Autodesk Inventor part; units mm, degrees
ref_plane "YZ Plane" through (0, 0, 0) normal (1, 0, 0) x (0, 1, 0)
ref_plane "XZ Plane" through (0, 0, 0) normal (0, 1, 0) x (-1, 0, 0)
ref_plane "XY Plane" through (0, 0, 0) normal (0, 0, 1) x (1, 0, 0)
sketch "Sketch1" plane through (0, 0, 0) normal (0, 0, 1) x (1, 0, 0)
  circle A0 centre (0, 0) radius 107.95
  circle A1 centre (0, 0) radius 114.3
  circle A2 centre (0, 0) radius 107.95
  circle A3 centre (0, 0) radius 107.95
  line L0 (-63.5, -63.5) -> (63.5, -63.5)
  line L1 (63.5, -63.5) -> (63.5, 63.5)
  line L2 (63.5, 63.5) -> (-63.5, 63.5)
  line L3 (-63.5, 63.5) -> (-63.5, -63.5)
  line L4 (-63.5, -63.5) -> (63.5, 63.5) construction
  line L5 (63.5, -63.5) -> (-63.5, 63.5) construction
  line L6 (57.15, 57.15) -> (57.15, -57.15)
  line L7 (57.15, -57.15) -> (-57.15, -57.15)
  line L8 (-57.15, -57.15) -> (-57.15, 57.15)
  line L9 (-57.15, 57.15) -> (57.15, 57.15)
  dimension "d0" = 127
  dimension "d1" = 127
  dimension "d2" = 6.35
extrude "Extrusion1" add sketch "Sketch1" along normal blind 6.35 contours L3 L2 L1 L0 | L6 L7 L8 L9
sketch "Sketch2" plane through (0, 0, 6.35) normal (0, 0, 1) x (1, 0, 0)
  line L0 (63.5, -63.5) -> (63.5, 63.5)
  line L1 (-63.5, 63.5) -> (63.5, 63.5)
  line L2 (63.5, 63.5) -> (63.5, -63.5)
  line L3 (63.5, -63.5) -> (-63.5, -63.5)
  line L4 (-63.5, -63.5) -> (-63.5, 63.5)
  line L5 (-63.5, 63.5) -> (63.5, -63.5) construction
  line L6 (63.5, 63.5) -> (-63.5, -63.5) construction
  line L7 (-57.15, -57.15) -> (57.15, -57.15)
  line L8 (57.15, -57.15) -> (57.15, 57.15)
  line L9 (57.15, 57.15) -> (-57.15, 57.15)
  line L10 (-57.15, 57.15) -> (-57.15, -57.15)
  point P0 (0, 0)
  dimension "d5" = 6.35
extrude "Extrusion2" add sketch "Sketch2" along normal blind 152.4
sketch "Sketch3" plane through (-63.5, -63.5, 0) normal (-1, 0, 0) x (0, 0, 1)
  line L0 (0, 127) -> (0, 0)
  line L1 (0, 0) -> (158.75, 0)
  line L2 (158.75, 127) -> (158.75, 0)
  line L3 (0, 127) -> (158.75, 127)
  point P0 (0, 63.5)
extrude "Extrusion3" add sketch "Sketch3" along normal blind 19.05
sketch "Sketch4" plane through (-82.55, -63.5, 0) normal (-1, 0, 0) x (0, 0, 1)
  line L0 (107.95, 6.35) -> (146.05, 6.35)
  line L1 (146.05, 6.35) -> (146.05, 120.65)
  line L2 (146.05, 120.65) -> (107.95, 120.65)
  line L3 (107.95, 120.65) -> (107.95, 6.35)
  line L4 (107.95, 6.35) -> (146.05, 120.65) construction
  line L5 (146.05, 6.35) -> (107.95, 120.65) construction
  line L6 (158.75, 127) -> (0, 127)
  line L7 (0, 0) -> (158.75, 0)
  line L8 (158.75, 0) -> (158.75, 127)
  point P0 (0, 63.5)
  point P1 (127, 63.5)
  dimension "d10" = 38.1
  dimension "d11" = 114.3
  dimension "d12" = 6.35
  dimension "d13" = 6.35
  dimension "d14" = 12.7
extrude "Extrusion4" cut sketch "Sketch4" against normal blind 7.62
ref_plane "Work Plane1" through (0, 0, 25.4) normal (0, 0, 1) x (1, 0, 0)
sketch "Sketch6" plane through (0, 0, 25.4) normal (0, 0, 1) x (1, 0, 0)
  line L0 (-57.15, -57.15) -> (57.15, -57.15)
  line L1 (57.15, -57.15) -> (57.15, 57.15)
  line L2 (57.15, 57.15) -> (-57.15, 57.15)
  line L3 (-57.15, 57.15) -> (-57.15, -57.15)
  point P0 (0, 0)
extrude "Extrusion5" add sketch "Sketch6" along normal blind 6.35
sketch "Sketch7" plane through (63.5, 63.5, 158.75) normal (0, 1, 0) x (1, 0, 0)
  line L0 (-6.35, 133.35) -> (-120.65, 133.35)
  line L1 (-120.65, 127) -> (-6.35, 127)
  circle A0 centre (-19.05, 122.0738) radius 3.175
  circle A1 centre (-43.18, 122.0738) radius 3.175
  circle A2 centre (-67.31, 122.0738) radius 3.175
  circle A3 centre (-91.44, 122.0738) radius 3.175
  circle A4 centre (-115.57, 122.0738) radius 3.175
  line L2 (-15.875, 122.0738) -> (-22.225, 122.0738)
  line L3 (-40.005, 122.0738) -> (-46.355, 122.0738)
  line L4 (-64.135, 122.0738) -> (-70.485, 122.0738)
  line L5 (-88.265, 122.0738) -> (-94.615, 122.0738)
  line L6 (-112.395, 122.0738) -> (-118.745, 122.0738)
  point P0 (-63.5, 158.75)
  dimension "d20" = 6.35
  dimension "d21" = 12.7
  dimension "d24" = 24.13
extrude "Extrusion6" cut sketch "Sketch7" against normal blind 127 contours L2 A0 | L3 A1 | L4 A2 | L5 A3 | L6 A4 picked at (-18.2578, 122.7756) picked at (-43.0524, 123.1244) picked at (-66.7088, 122.9448) picked at (-90.8388, 122.9448) picked at (-114.8476, 123.4366)
sketch "Sketch8" plane through (63.5, -63.5, 0) normal (1, 0, 0) x (0, 0, -1)
  line L0 (-6.35, 120.65) -> (-25.4, 120.65)
  line L1 (-158.75, 6.35) -> (-6.35, 6.35)
  line L2 (-6.35, 120.65) -> (-158.75, 120.65)
  line L3 (-6.35, 120.65) -> (-6.35, 6.35)
  line L4 (-6.35, 6.35) -> (-6.35, 120.65)
  line L5 (-28.575, 6.35) -> (-28.575, 120.65)
  point P0 (0, 63.5)
  point P1 (-25.4, 6.35)
extrude "Extrusion7" cut sketch "Sketch8" against normal blind 6.35
sketch "Sketch9" plane through (-57.15, 57.15, 6.35) normal (0, -1, 0) x (1, 0, 0)
  circle A0 centre (117.475, 19.05) radius 2.033
  line L0 (114.3, 19.05) -> (0, 19.05)
  line L1 (0, 0) -> (0, 19.05)
  line L2 (120.65, 0) -> (0, 0)
  line L3 (120.65, 22.225) -> (120.65, 0)
  line L4 (120.65, 22.225) -> (114.3, 22.225)
  line L5 (114.3, 22.225) -> (114.3, 19.05)
  point P0 (57.15, -6.35)
  dimension "d34" = 3.175
  dimension "d35" = 3.175
extrude "Extrusion8" cut sketch "Sketch9" along normal mid plane 254 contours A0
sketch "Sketch10" plane through (0, 0, 0) normal (0, 0, -1) x (-1, 0, 0)
  line L0 (57.15, 57.15) -> (57.15, -57.15)
  line L1 (74.93, -57.15) -> (74.93, 57.15)
  line L2 (57.15, 57.15) -> (74.93, 57.15)
  line L3 (82.55, -57.15) -> (74.93, -57.15)
  line L4 (57.15, -57.15) -> (74.93, -57.15)
  line L5 (60.325, 57.15) -> (60.325, -57.15)
  point P0 (0, 0)
  dimension "d40" = 3.175
extrude "Extrusion9" cut sketch "Sketch10" against normal blind 114.3 contours L2 L1 L4 L5
sketch "Sketch11" plane through (-82.55, -63.5, 0) normal (-1, 0, 0) x (0, 0, 1)
  line L0 (6.35, 120.65) -> (6.35, 6.35)
  line L1 (6.35, 120.65) -> (6.35, 6.35)
  line L2 (25.4, 120.65) -> (25.4, 6.35)
  line L3 (6.35, 6.35) -> (25.4, 6.35)
  line L4 (6.35, 120.65) -> (25.4, 120.65)
  line L5 (25.4, 120.65) -> (6.35, 120.65)
  point P0 (0, 63.5)
extrude "Extrusion10" cut sketch "Sketch11" against normal blind 42.8625
sketch "Sketch12" plane through (-60.325, -57.15, 0) normal (-1, 0, 0) x (0, 0, 1)
  point P0 (0, 57.15)
sketch "Sketch13" plane through (-60.325, -57.15, 0) normal (-1, 0, 0) x (0, 0, 1)
  line L0 (0, 114.3) -> (6.35, 114.3)
  line L1 (6.35, 114.3) -> (0, 114.3)
  line L2 (0, 114.3) -> (0, -0.7007)
  line L3 (0, 120.65) -> (0, -6.35)
  line L4 (0, 0) -> (6.35, 0)
  line L5 (6.35, 0) -> (6.35, 114.3)
  point P0 (0, 57.15)
extrude "Extrusion11" add sketch "Sketch13" along normal blind 22.225
sketch "Sketch14" plane through (-82.55, -57.15, 25.4) normal (0, 0, -1) x (-1, 0, 0)
  line L0 (0, 114.3) -> (0, 0)
  line L1 (0, 114.3) -> (-7.62, 114.3)
  line L2 (0, 114.3) -> (-7.62, 114.3)
  line L3 (-7.62, 0) -> (-7.62, 114.3)
  line L4 (-7.62, 114.3) -> (-7.62, 0)
  line L5 (0, 0) -> (-7.62, 0)
  line L6 (-7.62, 0) -> (0, 0)
  line L7 (0, 0) -> (0, 114.3)
  point P0 (-82.55, 57.15)
extrude "Extrusion12" add sketch "Sketch14" along normal blind 22.225
sketch "Sketch16" plane through (63.5, 63.5, 158.75) normal (0, 1, 0) x (1, 0, 0)
  line L0 (-138.43, 152.4) -> (-138.43, 50.8)
  line L1 (-138.43, 58.9187) -> (-142.4244, 58.9187)
  line L2 (-142.4244, 58.9187) -> (-142.4244, 64.1535)
  line L3 (-142.4244, 64.1535) -> (-146.05, 64.1535)
  line L4 (-146.05, 158.75) -> (-146.05, 0)
  line L5 (-146.05, 150.6067) -> (-137.3483, 150.6067)
  line L6 (-137.3483, 150.6067) -> (-137.3483, 58.9187)
  line L7 (-137.3483, 58.9187) -> (-138.43, 58.9187)
  point P0 (-63.5, 158.75)
  point P1 (-138.43, 150.6067)
extrude "Extrusion13" cut sketch "Sketch16" against normal blind 122.2375 contours L0 L1 L2 L3 L4 L5
sketch "Sketch17" plane through (63.5, 63.5, 158.75) normal (0, 1, 0) x (1, 0, 0)
  line L0 (-138.43, 150.6067) -> (-138.43, 154.3098)
  line L1 (-138.43, 154.3098) -> (-141.7479, 154.3098)
  line L2 (-141.7479, 154.3098) -> (-141.7479, 150.6067)
  line L3 (-146.05, 150.6067) -> (-138.43, 150.6067)
  point P0 (-63.5, 158.75)
extrude "Extrusion14" cut sketch "Sketch17" against normal blind 122.2375
sketch "Sketch19" plane through (-60.325, -57.15, 25.4) normal (-1, 0, 0) x (0, 0, 1)
  line L0 (10.614, 53.34) -> (11.249, 53.34)
  line L1 (11.249, 53.34) -> (11.249, 45.72)
  line L2 (11.249, 45.72) -> (10.614, 45.72)
  line L3 (10.614, 45.72) -> (10.614, 53.34)
  line L4 (10.614, 60.9551) -> (11.249, 60.9551)
  line L5 (11.249, 60.9551) -> (11.249, 68.5751)
  line L6 (11.249, 68.5751) -> (10.614, 68.5751)
  line L7 (10.614, 68.5751) -> (10.614, 60.9551)
  point P0 (-25.4, 57.15)
  dimension "d53" = 0.635
  dimension "d54" = 7.62
  dimension "d55" = 0.635
  dimension "d56" = 7.62
  dimension "d57" = 0.635
extrude "Extrusion15" cut sketch "Sketch19" against normal blind 47.625
properties part number "SqPot"
Can you work these out from the model? Positions are in its coordinate system, mm. A direction names the side the tool comes from. Coordinates: 2 decimals unless noted, no trailing zeros. Order: outer loops, then holes, each group sorted by start corner. A loop starts at its lowest first (then second) coordinate and runs counter-clockwise, first axis right, second up.
1. If we section it at D-D (x = -66): Please give me the cut outline in (y, z), then the cut area to 3 significant figures.
2. If we section it at B-B (z = 135): Please give me the cut outline in (x, y).
3. I'm going to push flat-ended pins straight in: pin 1 (1.5 mm diameter, centred on x = -0.5, y = -1.5, fed in from +Z); pin 2 (1 mm diameter, centred on x = -58, y = -8.5, fed in from -Z); pin 3 (1.6 mm diameter, centred on y = -27.5, z = 27, fed in from +X); pin 4 (12 mm diameter, centred on y = -31.5, z = 72, fed in from -X) (3 decimals). Where does each tip first touch, or does it pass through?
4. If we section it at C-C (y = 8.5): Give the number of separate pieces and of enclosed holes in the cut face, then the cut area to 3 significant figures.
5. I need wall thicknesses on line 1 (X direction, y = -45, z = 99) (3 decimals); line 2 (Z direction, x = -4, y = -54); line 3 (X direction, y = -34, z = 134). Which ranges of each line are inside material? Lowest first, please.
6. For faces 1 (the face through (-79, -1, 146.05)), 2 (the face through (1, 57.15, 94)), 3 (the face through (-74.93, 30, 6)), which set-ups out of +Z, -Z, +X, -X, +Y, -Y let a thin tool reach every point of the face, with its end or its side?
7. Thinking about a two-plate mould opening in Z: for faces 4 (the face through (-9, -63.5, 78)), 5 (the face through (-52, 60, 36.676)), 6 (the face through (-58, -4, 158.75)), 7 (the face through (-27.9, 60.4, 33.5)), which applies, +Z half, -Z half, draft (parallel to the pull), parting line (faces both ways), or undercut?
8. If we section it at A-A (x = -27.94): Please give me the cut outline in (y, z), then the cut area to 3 significant figures.
Entries:
1. outline: (-63.5, 0) - (63.5, 0) - (63.5, 158.75) - (-63.5, 158.75) - close; hole (-57.15, 6.35) - (57.15, 6.35) - (57.15, 114.3) - (-57.15, 114.3) - close
1. area: 7,820 mm2
2. outline: (-82.55, -63.5) - (63.5, -63.5) - (63.5, 63.5) - (-82.55, 63.5) - (-82.55, 57.15) - (-74.93, 57.15) - (-74.93, -57.15) - (-82.55, -57.15) - close; hole (-57.15, -57.15) - (57.15, -57.15) - (57.15, 57.15) - (-57.15, 57.15) - close
3. pin 1: stops at z = 31.75
3. pin 2: stops at z = 0
3. pin 3: stops at x = 57.15
3. pin 4: stops at x = -60.325
4. separate pieces: 4
4. enclosed holes: 0
4. area: 3,730 mm2
5. line 1: x = -82.55 to -78.924, -60.325 to -57.15, 57.15 to 63.5
5. line 2: z = 0 to 6.35, 25.4 to 31.75
5. line 3: x = -74.93 to -57.15, 57.15 to 63.5
6. face 1: -X
6. face 2: +Z
6. face 3: +Y
7. face 4: draft
7. face 5: undercut
7. face 6: +Z half
7. face 7: undercut
8. outline: (-63.5, 0) - (63.5, 0) - (63.5, 33.5) - (57.15, 33.5) - (57.15, 31.75) - (-57.15, 31.75) - (-57.15, 33.5) - (-63.5, 33.5) - close; (-63.5, 36.68) - (-57.15, 36.68) - (-57.15, 158.75) - (-63.5, 158.75) - close; (57.15, 36.68) - (63.5, 36.68) - (63.5, 158.75) - (57.15, 158.75) - close; hole (-57.15, 6.35) - (57.15, 6.35) - (57.15, 25.4) - (-57.15, 25.4) - close
8. area: 3,430 mm2
